from build123d import *

# Parameters (mm, degrees)
F0_R     = 100
F0_R_2   = 61
F1_DEPTH = 250
F0_R_3   = 19
F2_DEPTH = 170
F3_R     = 30
F3_R_2   = 19
F4_DEPTH = 25


with BuildPart() as f1:
    # F0 (on Front) → F1 (new body)
    with BuildSketch(Plane.XZ):
        Circle(F0_R)
        Circle(F0_R_2, mode=Mode.SUBTRACT)
    extrude(amount=F1_DEPTH)

    # F0 (on Front) → F2 (join)
    with BuildSketch(Plane.XZ):
        Circle(F0_R_2)
        Circle(F0_R_3, mode=Mode.SUBTRACT)
    extrude(amount=F2_DEPTH)

    # F3 (on face) → F4 (cut)
    with BuildSketch(Plane(origin=(0, 0, 0), x_dir=(-1, 0, 0), z_dir=(0, 1, 0))):
        Circle(F3_R)
        Circle(F3_R_2, mode=Mode.SUBTRACT)
    extrude(amount=-F4_DEPTH, mode=Mode.SUBTRACT)


solid = f1.part
Verification items for the finished model (mm, model axes). A direction names the side the tool comes from. Round coordinates to 2 decimals unless told otherwise and drop trailing zeros. Loops run counter-clockwise (first coordinate to the right, second up) from the corner with the lowest first, then second, coordinate; pieces in that order, holes last. Notation, with made-up numbers: (-7.5, 25.5) - (50.5, 25.5) arc R31 ccw to (50.5, 49.5) - close; hole circle Ø7 at (18, 50). An arc over 180 degrees is marked (long way). Use a Markdown table: item, result. Add a question column.
1. Access from +Z, -Z, +X, -X, +Y, -Y to the whole of each face (thin tool, end or side, straight path). Record for faces 1 (the face through (8.767, -96.485, -16.856)), 2 (the face through (12.7, -170, 14.4)), 3 (the face through (0, -25, -20)).
2. Section check D-D, the plane z = 35. Record the boundary of the cut face in (x, y), plus the area to 3 significant figures.
3. Gauge pin test, flat ends, axial feed: pin 1 (1.5 mm diameter, centred on x = -73, y = -59.5, fed in from +Z); pin 2 (1 mm diameter, centred on x = -23.5, z = -14, fed in from +Y); pin 3 (6 mm diameter, centred on x = 63.5, y = -37, fed in from -Z). Record the tip position at first contact, or that the pin passes through.
4. Release check for a two-part mould opening along X. For faces 4 (the face through (-46, -250, -43)), 5 (the face through (95.38, -123.25, 30.04)), 6 (the face through (-48.408, -209.44, -37.118)) record: released by +X, released by -X, zero draft, split by the parting line, or undercut.
5. Section check A-A, the plane z = 0. Record the boundary of the cut face in (x, y), plus the area to 3 significant figures.
6. Section check C-C, the plane y = -88.5. Record the boundary of the cut face in (x, z).
7. Thickness scan on probe 1 along Z at (x, y) = (0, -210.5); probe 2 along Z at (x, y) = (0, -5.25); probe 3 along Y at (x, z) = (-6, -32). Record the ranges inside material, lowest first. Write a range as [from, to].
8. Section check B-B, the plane x = 0. Record the boundary of the cut face in (y, z).
Checks:
| question | item | result |
|---|---|---|
| 1 | face 1 | +Y, -Y |
| 1 | face 2 | -Y |
| 1 | face 3 | +Y |
| 2 | outline | (-93.67, -250) - (-49.96, -250) - (-49.96, -170) - (49.96, -170) - (49.96, -250) - (93.67, -250) - (93.67, 0) - (-93.67, 0) - close |
| 2 | area | 38,800 mm^2 |
| 3 | pin 1 | stops at z = 69.14 |
| 3 | pin 2 | stops at y = -25 |
| 3 | pin 3 | stops at z = -79.62 |
| 4 | face 4 | zero draft |
| 4 | face 5 | split by the parting line |
| 4 | face 6 | undercut |
| 5 | outline | (-100, -250) - (-61, -250) - (-61, -170) - (-19, -170) - (-19, -25) - (-30, -25) - (-30, 0) - (-100, 0) - close; (19, -170) - (61, -170) - (61, -250) - (100, -250) - (100, 0) - (30, 0) - (30, -25) - (19, -25) - close |
| 5 | area | 33,200 mm^2 |
| 6 | outline | circle Ø200 at (0, 0); hole circle Ø38 at (0, 0) |
| 7 | probe 1 | z = [-100, -61], [61, 100] |
| 7 | probe 2 | z = [-100, -30], [30, 100] |
| 7 | probe 3 | y = [-170, 0] |
| 8 | outline | (-250, -100) - (0, -100) - (0, -30) - (-25, -30) - (-25, -19) - (-170, -19) - (-170, -61) - (-250, -61) - close; (-250, 61) - (-170, 61) - (-170, 19) - (-25, 19) - (-25, 30) - (0, 30) - (0, 100) - (-250, 100) - close |
